For this review, take the finished solid that the model builds, in its own axes (mm). Face numbers are marked on the shaded views. A direction names the side the tool comes from. Round coordinates to 2 decimals unless told otherwise and drop trailing zeros. Order: outer loops, then holes, each group sorted by start corner. A loop starts at its lowest first (then second) coordinate and runs counter-clockwise, first axis right, second up.
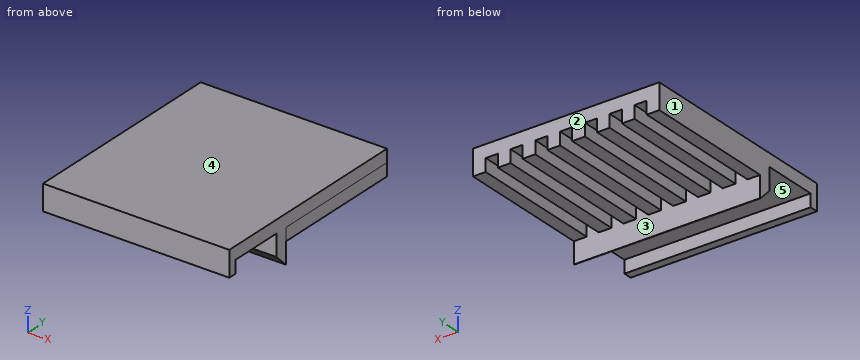
from build123d import *

# Parameters (mm, degrees)
BOX_W                  = 44
BOX_H                  = 48
BOX_DEPTH              = 3
BOX001_W               = 44
BOX001_H               = 2
BOX001_DEPTH           = 6
BOX002_W               = 44
BOX002_H               = 3
BOX002_DEPTH           = 8
CHAMFER_SIZE           = 2.9
BOX003_W               = 3
BOX003_H               = 32
BOX003_DEPTH           = 3
LINEARPATTERN001_COUNT = 8
LINEARPATTERN001_PITCH = 5.857143


with BuildPart() as part:
    # Box → Box (join)
    with BuildSketch(Plane.XY):
        with Locations((22, 24)):
            Rectangle(BOX_W, BOX_H)
    extrude(amount=BOX_DEPTH)

    # Box001 → Box001 (join)
    with BuildSketch(Plane(origin=(0, -2, -3), x_dir=(1, 0, 0), z_dir=(0, 0, 1))):
        with Locations((22, 1)):
            Rectangle(BOX001_W, BOX001_H)
    extrude(amount=BOX001_DEPTH)

    # Box002 → Box002 (join)
    with BuildSketch(Plane(origin=(0, 13, -8), x_dir=(1, 0, 0), z_dir=(0, 0, 1))):
        with Locations((22, 1.5)):
            Rectangle(BOX002_W, BOX002_H)
    extrude(amount=BOX002_DEPTH)

    # Chamfer
    chamfer_edges = [part.edges().sort_by_distance(p)[0] for p in [
        (22, 13, -8),
    ]]
    chamfer(chamfer_edges, length=CHAMFER_SIZE)

    # Box003 → Box003 (join)
    with BuildSketch(Plane(origin=(0, 16, -3), x_dir=(1, 0, 0), z_dir=(0, 0, 1))):
        with Locations((1.5, 16)):
            Rectangle(BOX003_W, BOX003_H)
    box003 = extrude(amount=BOX003_DEPTH)

    # LinearPattern001: Box003 ×8
    with Locations(*[(i * LINEARPATTERN001_PITCH, 0, 0) for i in range(1, LINEARPATTERN001_COUNT)]):
        add(box003)


solid = part.part
(1) Tool access review of the marked faces 4 and 5: name each direction out of +Z, -Z, +X, -X, +Y, -Y from which nothing blocks a thin tool from reaching the whole face with its end or side.
(2) Draft analysis for pull direction X (two halves, no side actions). For the marked faces 1, 2 and 3, state which applies: pulls with the +X half, pulls with the -X half, needs draft (parallel to the pull), parting line crosses it, or undercut.
(3) Wall thickness on L1, parallel to Y at x = 32, z = -0.75; L2, parallel to Z at x = 29.5, y = 35.5; L3, parallel to Z at x = 25.5, y = 7.5: over which ranges is each line inside the solid? List them lowest first.
(4) Add section D-D on y = 9. Give the boundary of the cut face in (x, z), plus the area to 3 significant figures.
(5) Add section B-B on x = 11. Give the boundary of the cut face in (y, z), plus the area to 3 significant figures.
(6) Add section C-C on x = 30.5. Give the boundary of the cut face in (y, z), plus the area to 3 significant figures.
(7) Clearance check with flat-ended pins moving along their axes: P1, Ø4, axis at x = 13, z = -3.5, coming from the -Y side; P2, Ø3, axis at x = 14, y = 41.5, coming from the -Z side; P3, Ø0.9, axis at x = 33.5, y = 27.5, coming from the -Z side. State where each tip first meets the part, or that it passes through.
Here are the results:
1. face 4: +Z, +X, -X, +Y, -Y
1. face 5: -Z, +X, -X
2. face 1: pulls with the -X half
2. face 2: needs draft
2. face 3: undercut
3. L1: y = -2 to 0, 13 to 48
3. L2: z = -3 to 3
3. L3: z = 0 to 3
4. outline: (0, 0) - (44, 0) - (44, 3) - (0, 3) - close
4. area: 132 mm2
5. outline: (-2, -3) - (0, -3) - (0, 0) - (13, 0) - (13, -5.1) - (15.9, -8) - (16, -8) - (16, 0) - (48, 0) - (48, 3) - (-2, 3) - close
5. area: 176 mm2
6. outline: (-2, -3) - (0, -3) - (0, 0) - (13, 0) - (13, -5.1) - (15.9, -8) - (16, -8) - (16, -3) - (48, -3) - (48, 3) - (-2, 3) - close
6. area: 272 mm2
7. P1: stops at y = -2
7. P2: stops at z = -3
7. P3: stops at z = 0
